Here's how the part is built. I have some questions about the finished solid (model axes, mm). A direction names the side the tool comes from. Give positions to 0.01 mm unless a question says otherwise; leave off trailing zeros. Write each loop counter-clockwise with the first axis right and the second up, starting at its lowest first coordinate (ties: lowest second). Pieces come first, ordered by that corner, then holes. Notation, with made-up numbers: M -20,36 L -16,36 A31 cw -16,62 Z; hole C 57,12.25 d7. An arc over 180 degrees is marked long. Answer as CSV lines item,"result". Start each with the question number.
Q1. For pin 1 (4 mm diameter, centred on y = 17, z = -3.5, fed in from -X); pin 2 (3.5 mm diameter, centred on x = 0, z = 0, fed in from +Y); pin 3 (4.5 mm diameter, centred on x = 0, z = 0, fed in from +Y), each with a flat end and sliding along its axis, tell me the tip position at first contact or that it passes through.
Q2. Thinking about a two-plate mould opening in X: for faces 3 (the flat face through (2.2, 20, 2.2)), 4 (the cylindrical face through (0, 10, 5)), 5 (the cylindrical face through (1.5, 4.44, -0.07)), which applies, +X half, -X half, draft (parallel to the pull), parting line (faces both ways), or undercut?
Q3. On a 3-axis mill with a long thin cutter (end or side, diameter ignored), from which of +Z, -Z, +X, -X, +Y, -Y can I reach the whole of each face in a straight line? I mean faces 1 (the flat face through (1.2, 0, 1.2)), 2 (the cylindrical face through (-0.596, 14.93, -2.685)). Say none if no direction works.
Q4. Suppose I cut it at D-D (y = 3.25). Write out the boundary of the cut face in (x, z).
Q5. Suppose I cut it at C-C (z = -4.5). Write out the boundary of the cut face in (x, y).
Q6. Suppose I cut it at B-B (y = 16.25). Write out the boundary of the cut face in (x, z).
Q7. If I drill on line 1 along Z through (x, y) = (0, 16.5); line 2 along Z through (x, y) = (0, 5), over which ranges is the centre line in solid material (lowest first)?
Autodesk Inventor part; units mm, degrees
ref_plane "YZ Plane" through (0, 0, 0) normal (1, 0, 0) x (0, 1, 0)
ref_plane "XZ Plane" through (0, 0, 0) normal (0, 1, 0) x (-1, 0, 0)
ref_plane "XY Plane" through (0, 0, 0) normal (0, 0, 1) x (1, 0, 0)
sketch "Sketch1" plane through (0, 0, 0) normal (0, 1, 0) x (-1, 0, 0)
  circle A0 centre (0, 0) radius 5
  circle A1 centre (0, 0) radius 1.5
  dimension "d0" = 10
  dimension "d1" = 3
extrude "Extrusion1" add sketch "Sketch1" along normal blind 10
sketch "Sketch2" plane through (0, 10, 0) normal (0, 1, 0) x (1, 0, 0)
  circle A0 centre (0, 0) radius 2.75
  circle A1 centre (0, 0) radius 5
  dimension "d4" = 5.5
extrude "Extrusion2" add sketch "Sketch2" along normal blind 10
thread "Thread1"
fillet "Fillet1" radius 1 1 edges at (1.5, 10, 0)
thread "Thread3"
properties part number "platform_adapter"
Resolved:
1,pin 1,"x = -4.77"
1,pin 2,"y = 9.66"
1,pin 3,"y = 9.97"
2,face 3,"draft"
2,face 4,"parting line"
2,face 5,"undercut"
3,face 1,"+Z, -Z, +X, -X, -Y"
3,face 2,"+Y"
4,outline,"C 0,0 d10; hole C 0,0 d3"
5,outline,"M -2.18,0 L 2.18,0 L 2.18,20 L -2.18,20 Z"
6,outline,"C 0,0 d10; hole C 0,0 d5.5"
7,line 1,"-5 to -2.75, 2.75 to 5"
7,line 2,"-5 to -1.5, 1.5 to 5"
